Part model, mm, in its own coordinate system. A direction names the side the tool comes from. Round coordinates to 2 decimals unless told otherwise and drop trailing zeros. Write each loop counter-clockwise with the first axis right and the second up, starting at its lowest first coordinate (ties: lowest second). Pieces come first, ordered by that corner, then holes. Notation, with made-up numbers: (56.5, 76.25) -> (105.5, 76.25) arc R20 ccw to (105.5, 84.25) -> close; hole circle Ø8 at (59, 7). An arc over 180 degrees is marked (long way). Return JSON: item names as keys, results as strings. Group by question number.
(1) Saw through at B-B (z = 4). List the corners of the cut face in (x, y), plus the area to 3 significant figures.
(2) Mould opens along Z. For faces 3 (the conical face through (-6.54, 1.01, -4.03)), 4 (the cylindrical face through (58.289, 1.239, -7.068)), 5 (the flat face through (-9, 7, 34)) say: +Z half, -Z half, draft (parallel to the pull), parting line (faces both ways), or undercut.
(3) Tool access for faces 1 (the flat face through (24, -4.5, 16)), 2 (the cylindrical face through (58.515, 1.239, 37.349)): list every direction of +Z, -Z, +X, -X, +Y, -Y with a clear straight run to the whole face (end or side of a thin tool).
(4) Saw through at A-A (x = 11). List the corners of the cut face in (y, z).
(5) Drop flat-ended pins along their axis: pin 1 Ø3 at (x, z) = (19, 31.5) entering from +Y; pin 2 Ø3 at (x, y) = (7, 2.5) entering from +Z; pin 3 Ø2.5 at (x, z) = (-6.64, -4.36) entering from +Y. Give the stop position or say it passes through.
(6) Drill centre lines: L1, parallel to X at y = 2.5, z = 35.5; L2, parallel to X at y = 5.75, z = 34.5; L3, parallel to Y at x = 41, z = 10.5. Where is each one in solid material? Low to high. Write a range as from..to.
Autodesk Inventor part; units mm, degrees
ref_plane "YZ Plane" through (0, 0, 0) normal (1, 0, 0) x (0, 1, 0)
ref_plane "XZ Plane" through (0, 0, 0) normal (0, 1, 0) x (-1, 0, 0)
ref_plane "XY Plane" through (0, 0, 0) normal (0, 0, 1) x (1, 0, 0)
sketch "proto-board hole layout" plane through (0, 0, 0) normal (0, 1, 0) x (-1, 0, 0)
  circle A0 centre (6.6395, -4.3647) radius 1.49
  circle A1 centre (-55.3405, -4.3647) radius 1.49
  circle A2 centre (-55.3405, 34.9153) radius 1.49
  circle A3 centre (6.6395, 34.9153) radius 1.49
  line L0 (5.1495, -4.3647) -> (-53.8505, -4.3647) construction
  line L1 (5.1495, 34.9153) -> (-53.8505, 34.9153) construction
  line L2 (-55.3405, 33.4253) -> (-55.3405, -2.8747) construction
  line L3 (6.6395, 33.4253) -> (6.6395, -2.8747) construction
  dimension "d0" = 2.98
  dimension "d1" = 59
  dimension "d2" = 36.3
sketch "Sketch3" plane through (0, 0, 0) normal (0, 1, 0) x (-1, 0, 0)
  circle A0 centre (6.6395, -4.3647) radius 1.49
  circle A1 centre (6.6395, -4.3647) radius 4
  point P0 (0, 0)
  dimension "d15" = 8
extrude "Extrusion2" add sketch "Sketch3" along normal blind 7 contours A0 | A1
sketch "Sketch4" plane through (-6.6395, 7, -4.3647) normal (0, 1, 0) x (1, 0, 0)
  circle A0 centre (0, 0) radius 4 construction
  point P0 (6.6395, -4.3647)
hole "Hole1" at (-6.6395, 7, -4.3647) direction (0, -1, 0) diameter 4 depth 5 tip angle 118
chamfer "Chamfer1" distance 1 distance2 2 1 edges at (-2.6395, 7, -4.3647) measured on face at (-9.9293, 7, -4.7642)
pattern_sketch "Sketch Driven Pattern1" from (-6.6395, 0, -4.3647) copies at (55.3405, 0, -4.3647) at (55.3405, 0, 34.9153) at (-6.6395, 0, 34.9153)
sketch "Sketch5" plane through (-6.6395, 0, 34.9153) normal (0, -1, 0) x (1, 0, 0)
  circle A0 centre (0, 0) radius 4
  circle A1 centre (61.98, 0) radius 4
  circle A2 centre (61.98, -39.28) radius 4
  circle A3 centre (0, -39.28) radius 4
  line L0 (-4, 4) -> (65.98, 4)
  line L1 (65.98, 4) -> (65.98, -43.28)
  line L2 (65.98, -43.28) -> (-4, -43.28)
  line L3 (-4, -43.28) -> (-4, 4)
  point P0 (6.6395, -34.9153)
  point P1 (-4, 0)
  point P2 (-4, -39.28)
  point P3 (0, -43.28)
  point P4 (61.98, -43.28)
  point P5 (65.98, -39.28)
  point P6 (65.98, 0)
  point P7 (61.98, 4)
  point P8 (0, 4)
extrude "Extrusion3" add sketch "Sketch5" along normal blind 4.5 contours A0 | A0 L0 A1 L1 A2 L2 A3 L3 | A1 | A3 | A2
properties part number "proto-board_standoffs_plate"
Computed values:
{
 "1": {"outline": "(-10.64, -4.5) -> (59.34, -4.5) -> (59.34, 0) -> (-10.64, 0) -> close", "area": "315 mm2"},
 "2": {"face 3": "undercut", "face 4": "undercut", "face 5": "draft"},
 "3": {"face 1": "+Z, -Z, +X, -X, -Y", "face 2": "+Y"},
 "4": {"outline": "(-4.5, -8.36) -> (0, -8.36) -> (0, 38.92) -> (-4.5, 38.92) -> close"},
 "5": {"pin 1": "y = 0", "pin 2": "through", "pin 3": "y = 1.55"},
 "6": {"L1": "-10.6..-8.55, -4.73..-2.68, 51.38..53.43, 57.25..59.3", "L2": "-10.24..-8.6, -4.68..-3.04, 51.74..53.38, 57.3..58.94", "L3": "-4.5..0"}
}
